```python
from build123d import *

# Parameters (mm, degrees)
CYLINDER_R          = 21.7805
CYLINDER_DEPTH      = 76.2
CYLINDER_ROLL_ANGLE = 90
SKETCH_R            = 16.7005
POCKET_DEPTH        = 76.2
SKETCH001_R         = 22.225
POCKET001_DEPTH     = 8.89
SKETCH002_R         = 22.225
POCKET002_DEPTH     = 8.89


with BuildPart() as part:
    # Cylinder → Cylinder (new body)
    with BuildSketch(Plane.XY):
        Circle(CYLINDER_R)
    extrude(amount=CYLINDER_DEPTH)


with BuildPart() as part_1:
    # Cylinder roll: moved
    add(part.part.rotate(Axis((0, 0, 0), (1, 0, 0)), CYLINDER_ROLL_ANGLE))


with BuildPart() as part_2:
    # Cylinder placement: moved
    add(part_1.part)

    # Sketch → Pocket (cut)
    with BuildSketch(Plane(origin=(0, 0, 0), x_dir=(1, 0, 0), z_dir=(0, 1, 0))):
        Circle(SKETCH_R)
    extrude(amount=-POCKET_DEPTH, mode=Mode.SUBTRACT)

    # Sketch001 → Pocket001 (cut)
    with BuildSketch(Plane(origin=(0, 0, 0), x_dir=(1, 0, 0), z_dir=(0, 1, 0))):
        Circle(SKETCH001_R)
        Polygon((-19.05, -10.998523), (-19.05, 10.998523), (0, 21.997045), (19.05, 10.998523), (19.05, -10.998523), (0, -21.997045), align=None, mode=Mode.SUBTRACT)
    extrude(amount=-POCKET001_DEPTH, mode=Mode.SUBTRACT)

    # Sketch002 → Pocket002 (cut)
    with BuildSketch(Plane.XZ.offset(76.2)):
        Circle(SKETCH002_R)
        Polygon((-19.05, -10.998523), (-19.05, 10.998523), (0, 21.997045), (19.05, 10.998523), (19.05, -10.998523), (0, -21.997045), align=None, mode=Mode.SUBTRACT)
    extrude(amount=-POCKET002_DEPTH, mode=Mode.SUBTRACT)


solid = part_2.part
```
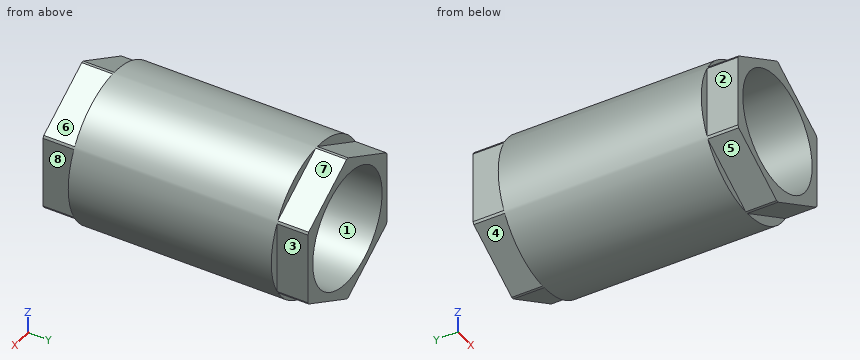
Model file for the job. Use its own axes, mm. Face numbers are marked on the shaded views. A direction names the side the tool comes from. Coordinates: 2 decimals unless noted, no trailing zeros. Loops run counter-clockwise (first coordinate to the right, second up) from the corner with the lowest first, then second, coordinate; pieces in that order, holes last. Notation, with made-up numbers: (15, 18.25) -> (64, 18.25) arc R6 ccw to (64, 22.25) -> close; hole circle Ø11 at (58, -20.5). An arc over 180 degrees is marked (long way). Answer as a JSON object with one key per item and string values.
Q1. 3-axis set-ups, long thin cutter, end or side, ignore diameter. For the marked faces 4, 5, 6, 7 and 8: which of +Z, -Z, +X, -X, +Y, -Y reach the whole face in a straight line?
Report:
{"face 4": "-Z, -X, +Y", "face 5": "-Z, -X, -Y", "face 6": "+Z, +X, -Y", "face 7": "+Z, +X, +Y", "face 8": "+Z, -Z, +X, -Y"}
Q2. Cut at A-A (z = 0). List the corners of the cut face in (x, y).
Report:
{"outline": "(-21.78, -67.31) -> (-19.05, -67.31) -> (-19.05, -76.2) -> (-16.7, -76.2) -> (-16.7, 0) -> (-19.05, 0) -> (-19.05, -8.89) -> (-21.78, -8.89) -> close; (16.7, -76.2) -> (19.05, -76.2) -> (19.05, -67.31) -> (21.78, -67.31) -> (21.78, -8.89) -> (19.05, -8.89) -> (19.05, 0) -> (16.7, 0) -> close"}
Q3. Pull direction X, two halves, no side cores. Call the marked faces 1, 2 and 3: released by +X, released by -X, zero draft, split by the parting line, or undercut.
Report:
{"face 1": "undercut", "face 2": "released by -X", "face 3": "released by +X"}
Q4. Probe probe 1 along Z at (x, y) = (0, -25); probe 2 along Y at (x, z) = (20.5, -3.5); probe 3 along X at (y, z) = (-29, 4.5). List the from-to ranges inside material, lowest first.
Report:
{"probe 1": "z = -21.78 to -16.7, 16.7 to 21.78", "probe 2": "y = -67.31 to -8.89", "probe 3": "x = -21.31 to -16.08, 16.08 to 21.31"}
Q5. Cut at D-D (z = 18.5). List the corners of the cut face in (x, y), and give its area (3 significant figures).
Report:
{"outline": "(-11.5, -67.31) -> (-6.06, -67.31) -> (-6.06, -76.2) -> (6.06, -76.2) -> (6.06, -67.31) -> (11.5, -67.31) -> (11.5, -8.89) -> (6.06, -8.89) -> (6.06, 0) -> (-6.06, 0) -> (-6.06, -8.89) -> (-11.5, -8.89) -> close", "area": "1,560 mm2"}
Q6. Flat gauge pins, fed straight in: P1, Ø2, axis at x = 20, z = -2, coming from the +Y side; P2, Ø6, axis at x = 17, y = -39, coming from the -Z side (3 decimals); P3, Ø4, axis at x = -8.5, y = -49, coming from the -Z side; P4, Ø5, axis at x = -9.5, y = -65.5, coming from the +Z side (3 decimals). Where does each tip first touch, or does it go through?
Report:
{"P1": "stops at y = 0", "P2": "stops at z = -16.685", "P3": "stops at z = -20.79", "P4": "stops at z = 20.625"}
Q7. Cut at B-B (x = 11). List the corners of the cut face in (y, z), and give its area (3 significant figures).
Report:
{"outline": "(-76.2, -15.65) -> (-67.31, -15.65) -> (-67.31, -18.8) -> (-8.89, -18.8) -> (-8.89, -15.65) -> (0, -15.65) -> (0, -12.57) -> (-76.2, -12.57) -> close; (-76.2, 12.57) -> (0, 12.57) -> (0, 15.65) -> (-8.89, 15.65) -> (-8.89, 18.8) -> (-67.31, 18.8) -> (-67.31, 15.65) -> (-76.2, 15.65) -> close", "area": "838 mm2"}
Q8. Cut at C-C (y = -24.5). List the corners of the cut face in (x, z), and give its area (3 significant figures).
Report:
{"outline": "circle Ø43.56 at (0, 0); hole circle Ø33.4 at (0, 0)", "area": "614 mm2"}
